Check sheet for the modelled part. Datum: model origin and axes. Units: mm. Face numbers are marked on the shaded views. A direction names the side the tool comes from. Round coordinates to 2 decimals unless told otherwise and drop trailing zeros. Write each loop counter-clockwise with the first axis right and the second up, starting at its lowest first coordinate (ties: lowest second). Pieces come first, ordered by that corner, then holes. Notation, with made-up numbers: (-5.75, 44) -> (9.25, 44) arc R24 ccw to (9.25, 55) -> close; hole circle Ø6 at (-40, 44.5). An arc over 180 degrees is marked (long way). One line per item, written item: value.
Autodesk Inventor part; units mm, degrees
ref_plane "YZ Plane" through (0, 0, 0) normal (1, 0, 0) x (0, 1, 0)
ref_plane "XZ Plane" through (0, 0, 0) normal (0, 1, 0) x (-1, 0, 0)
ref_plane "XY Plane" through (0, 0, 0) normal (0, 0, 1) x (1, 0, 0)
sketch "草图1" plane through (0, 0, 0) normal (0, 0, 1) x (1, 0, 0)
  circle A0 centre (0, 0) radius 15
  dimension "d0" = 30
extrude "拉伸1" add sketch "草图1" along normal blind 2
sketch "草图2" plane through (0, 0, 2) normal (0, 0, 1) x (1, 0, 0)
  line L0 (5.7735, -10) -> (-5.7735, -10)
  line L1 (-5.7735, -10) -> (-11.547, 0)
  line L2 (-11.547, 0) -> (-5.7735, 10)
  line L3 (-5.7735, 10) -> (5.7735, 10)
  line L4 (5.7735, 10) -> (11.547, 0)
  line L5 (11.547, 0) -> (5.7735, -10)
  line L6 (0, 0) -> (0, 3.0227)
  point P0 (0, 10)
  dimension "d3" = 3.0227
  dimension "d4" = 20
extrude "拉伸2" add sketch "草图2" along normal blind 8
fillet "圆角1" radius 0.5 13 edges at (-5.7735, -10, 6) (5.7735, -10, 6) (11.547, 0, 6) (5.7735, 10, 6) (-5.7735, 10, 6) (-11.547, 0, 6) (-8.6603, 5, 10) (-8.6603, -5, 10) (0, 10, 10) (8.6603, 5, 10) (8.6603, -5, 10) (0, -10, 10) (-15, 0, 2)
sketch "草图3" plane through (0, 0, 0) normal (0, 0, -1) x (-1, 0, 0)
  circle A0 centre (0, 0) radius 5
  dimension "d8" = 10
extrude "拉伸3" add sketch "草图3" along normal blind 67
thread "螺纹1"
chamfer "倒角1" distance 0.5 angle 45 1 edges at (5, 0, -67)
properties part number "主动轮固定螺丝"
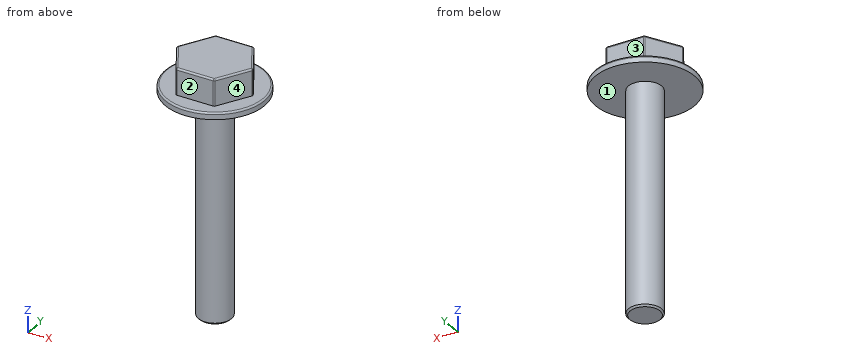
Item 1: Depth check by flat-ended pin: pin 1 (2 mm diameter, centred on x = -3, y = 7, fed in from -Z); pin 2 (6 mm diameter, centred on x = -1, z = 4.5, fed in from -Y); pin 3 (2 mm diameter, centred on x = 0.5, z = 5, fed in from +Y). Enter the tip coordinate at first touch or a pass-through.
Result set:
pin 1: z = 0
pin 2: y = -14.99
pin 3: y = 10
Item 2: Sectioned sample at A-A (x = 0). Enter the section's corners in (y, z).
Result set:
outline: (-15, 0) -> (-5, 0) -> (-5, -66.5) -> (-4.5, -67) -> (4.5, -67) -> (5, -66.5) -> (5, 0) -> (15, 0) -> (15, 1.5) arc R0.5 ccw to (14.5, 2) -> (10, 2) -> (10, 9.5) arc R0.5 ccw to (9.5, 10) -> (-9.5, 10) arc R0.5 ccw to (-10, 9.5) -> (-10, 2) -> (-14.5, 2) arc R0.5 ccw to (-15, 1.5) -> close
Item 3: Sectioned sample at B-B (z = -16). Enter the section's corners in (x, y), then the cut area to 3 significant figures.
Result set:
outline: circle Ø10 at (0, 0)
area: 78.5 mm^2
Item 4: Material ranges on line 1 along Z through (x, y) = (12, 4.25); line 2 along Y through (x, z) = (2.5, 5); line 3 along X through (y, z) = (-0.25, -27.5), recorded low to high.
Result set:
line 1: 0 to 2
line 2: -10 to 10
line 3: -4.99 to 4.99
Item 5: Tool access check on the marked faces 1, 2, 3 and 4. Record the directions out of +Z, -Z, +X, -X, +Y, -Y that give a thin tool (end or side, any length) a straight path to the whole face; none if there is none.
Result set:
face 1: -Z
face 2: +Z, +X, -X, -Y
face 3: +Z, +X, -X, +Y
face 4: +Z, +X, -Y
